from build123d import *

# Parameters (mm, degrees)
F0_W     = 482.6
F0_H     = 132.6
F1_DEPTH = 3
F2_W     = 3.5
F2_H     = 6.8
F3_W     = 3.5
F3_H     = 6.8
F4_W     = 3.5
F4_H     = 6.8
F5_W     = 3.5
F5_H     = 6.8
F6_DEPTH = 3
F7_R     = 38
F7_R_2   = 32
F7_R_3   = 1.6
F8_DEPTH = 3


with BuildPart() as f1:
    # F0 (on Front) → F1 (new body)
    with BuildSketch(Plane.XZ):
        Rectangle(F0_W, F0_H)
    extrude(amount=-F1_DEPTH)

    # F2 (on face) + F3 (on face) + F4 (on face) + F5 (on face) → F6 (cut)
    with BuildSketch(Plane.XZ):
        with Locations((-232.5, 28.6)):
            Rectangle(F2_W, F2_H)
        with BuildLine():
            Line((-230.75, 32), (-230.75, 25.2))
            ThreePointArc((-230.75, 25.2), (-227.35, 28.6), (-230.75, 32))
        make_face()
        with BuildLine():
            ThreePointArc((-234.25, 32), (-237.65, 28.6), (-234.25, 25.2))
            Line((-234.25, 25.2), (-234.25, 32))
        make_face()
    with BuildSketch(Plane.XZ):
        with Locations((-232.5, -28.6)):
            Rectangle(F3_W, F3_H)
        with BuildLine():
            Line((-230.75, -25.2), (-230.75, -32))
            ThreePointArc((-230.75, -32), (-227.35, -28.6), (-230.75, -25.2))
        make_face()
        with BuildLine():
            ThreePointArc((-234.25, -25.2), (-237.65, -28.6), (-234.25, -32))
            Line((-234.25, -32), (-234.25, -25.2))
        make_face()
    with BuildSketch(Plane.XZ):
        with Locations((232.5, 28.6)):
            Rectangle(F4_W, F4_H)
        with BuildLine():
            ThreePointArc((234.25, 25.2), (237.65, 28.6), (234.25, 32))
            Line((234.25, 32), (234.25, 25.2))
        make_face()
        with BuildLine():
            Line((230.75, 25.2), (230.75, 32))
            ThreePointArc((230.75, 32), (227.35, 28.6), (230.75, 25.2))
        make_face()
    with BuildSketch(Plane.XZ):
        with Locations((232.5, -28.6)):
            Rectangle(F5_W, F5_H)
        with BuildLine():
            Line((234.25, -25.2), (234.25, -32))
            ThreePointArc((234.25, -32), (237.65, -28.6), (234.25, -25.2))
        make_face()
        with BuildLine():
            ThreePointArc((230.75, -25.2), (227.35, -28.6), (230.75, -32))
            Line((230.75, -32), (230.75, -25.2))
        make_face()
    extrude(amount=-F6_DEPTH, mode=Mode.SUBTRACT)

    # F7 (on face) → F8 (cut)
    with BuildSketch(Plane.XZ):
        with Locations((-120.65, 0)):
            Circle(F7_R)
        with Locations((120.65, 0)):
            Circle(F7_R_2)
        Polygon((20.85, -0.5), (20.85, 6), (-20.85, 6), (-20.85, -0.5), (-16.75, -0.5), (-16.75, -6), (16.75, -6), (16.75, -0.5), align=None)
        with Locations((20.32, -5)):
            Circle(F7_R_3)
        with Locations((-20.32, -5)):
            Circle(F7_R_3)
    extrude(amount=-F8_DEPTH, mode=Mode.SUBTRACT)


solid = f1.part
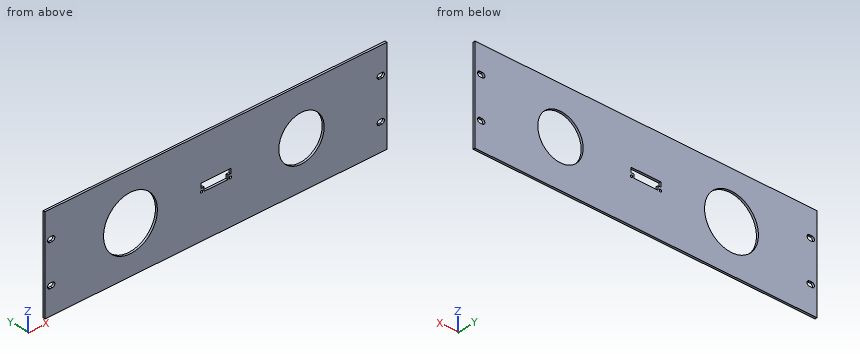
Source: CAD feature listing. Evaluate the final solid. Frame: model axes, mm. Round coordinates to 2 decimals unless told otherwise and drop trailing zeros. Write each loop counter-clockwise with the first axis right and the second up, starting at its lowest first coordinate (ties: lowest second). Pieces come first, ordered by that corner, then holes. Notation, with made-up numbers: (20, 52.5) - (45, 52.5) arc R17 ccw to (45, 64.5) - close; hole circle Ø9 at (17.25, -33). An arc over 180 degrees is marked (long way). Use CSV: the item, a comma, the result in double quotes. Start each with the question number.
(1) Cut plane B-B, the plane y = 0.45. Give the number of separate pieces and of enclosed holes in the cut face, and give its area (3 significant figures).
(2) Cut plane C-C, the plane x = -120.65. Return loops of the section in (y, z).
(3) Cut plane A-A, the plane x = 120.65. Return loops of the section in (y, z), and give its area (3 significant figures).
(4) Material intervals for probe 1 along Z at (x, y) = (20.32, 2); probe 2 along Z at (x, y) = (120.65, 0.8); probe 3 along X at (y, z) = (2.35, 15.5), sorted ascending. Write a range as [from, to].
Geometry says:
1,separate pieces,"1"
1,enclosed holes,"9"
1,area,"55,500 mm²"
2,outline,"(0, -66.3) - (3, -66.3) - (3, -38) - (0, -38) - close; (0, 38) - (3, 38) - (3, 66.3) - (0, 66.3) - close"
3,outline,"(0, -66.3) - (3, -66.3) - (3, -32) - (0, -32) - close; (0, 32) - (3, 32) - (3, 66.3) - (0, 66.3) - close"
3,area,"206 mm²"
4,probe 1,"[-66.3, -6.6], [-3.4, -0.5], [6, 66.3]"
4,probe 2,"[-66.3, -32], [32, 66.3]"
4,probe 3,"[-241.3, -155.35], [-85.95, 92.65], [148.65, 241.3]"
